Autodesk Inventor part; units mm, degrees
ref_plane "YZ Plane" through (0, 0, 0) normal (1, 0, 0) x (0, 1, 0)
ref_plane "XZ Plane" through (0, 0, 0) normal (0, 1, 0) x (-1, 0, 0)
ref_plane "XY Plane" through (0, 0, 0) normal (0, 0, 1) x (1, 0, 0)
sketch "Sketch1" plane through (0, 0, 0) normal (0, 0, 1) x (1, 0, 0)
  line L0 (-18.7833, 39.6114) -> (-18.7833, -39.6114)
  line L1 (-18.7833, -39.6114) -> (18.7833, -39.6114)
  line L2 (18.7833, -39.6114) -> (18.7833, 39.6114)
  line L3 (18.7833, 39.6114) -> (-18.7833, 39.6114)
  line L4 (-15.6083, 36.4364) -> (15.6083, 36.4364)
  line L5 (15.6083, 36.4364) -> (15.6083, -36.4364)
  line L6 (15.6083, -36.4364) -> (-15.6083, -36.4364)
  line L7 (-15.6083, -36.4364) -> (-15.6083, 36.4364)
  point P0 (0, 0)
extrude "Extrusion1" add sketch "Sketch1" along normal blind 3.175 contours L3 L2 L1 L0 | L4 L5 L6 L7
sketch "Sketch2" plane through (0, 0, 0) normal (0, 0, -1) x (-1, 0, 0)
  line L0 (-15.6083, -36.4364) -> (15.6083, -36.4364)
  line L1 (-15.6083, 36.4364) -> (-15.6083, -36.4364)
  line L2 (15.6083, 36.4364) -> (-15.6083, 36.4364)
  line L3 (15.6083, -36.4364) -> (15.6083, 36.4364)
  line L4 (-15.3543, 36.1824) -> (-15.3543, -36.1824)
  line L5 (-15.3543, -36.1824) -> (15.3543, -36.1824)
  line L6 (15.3543, -36.1824) -> (15.3543, 36.1824)
  line L7 (15.3543, 36.1824) -> (-15.3543, 36.1824)
  point P0 (0, 0)
  dimension "d2" = 0.254
extrude "Extrusion2" add sketch "Sketch2" along normal blind 1.5875 contours L7 L6 L5 L4
sketch "Sketch3" plane through (0, 0, -1.5875) normal (0, 0, -1) x (-1, 0, 0)
  line L0 (-15.3543, 36.1824) -> (-15.3543, -36.1824)
  line L1 (-15.3543, 36.1824) -> (-9.0043, 36.1824)
  line L2 (-9.0043, 36.1824) -> (-9.0043, 29.8324)
  line L3 (-9.0043, 29.8324) -> (-15.3543, 29.8324)
  line L4 (-15.3543, 29.8324) -> (-15.3543, 36.1824)
  line L5 (15.3543, 36.1824) -> (-15.3543, 36.1824)
  line L6 (15.3543, 36.1824) -> (9.0043, 36.1824)
  line L7 (9.0043, 36.1824) -> (9.0043, 29.8324)
  line L8 (9.0043, 29.8324) -> (15.3543, 29.8324)
  line L9 (15.3543, 29.8324) -> (15.3543, 36.1824)
  line L10 (-15.3543, -36.1824) -> (15.3543, -36.1824)
  line L11 (-15.3543, -36.1824) -> (-9.0043, -36.1824)
  line L12 (-9.0043, -36.1824) -> (-9.0043, -29.8324)
  line L13 (-9.0043, -29.8324) -> (-15.3543, -29.8324)
  line L14 (-15.3543, -29.8324) -> (-15.3543, -36.1824)
  line L15 (15.3543, 36.1824) -> (15.3543, -36.1824)
  line L16 (15.3543, -36.1824) -> (9.0043, -36.1824)
  line L17 (9.0043, -36.1824) -> (9.0043, -29.8324)
  line L18 (9.0043, -29.8324) -> (15.3543, -29.8324)
  line L19 (15.3543, -29.8324) -> (15.3543, -36.1824)
  point P0 (0, 0)
  dimension "d5" = 6.35
  dimension "d6" = 6.35
  dimension "d7" = 6.35
  dimension "d8" = 6.35
  dimension "d9" = 6.35
  dimension "d10" = 6.35
  dimension "d11" = 6.35
  dimension "d12" = 6.35
extrude "Extrusion3" add sketch "Sketch3" along normal blind 5.08 contours L1 L2 L3 L0 | L13 L12 L10 L0 | L5 L9 L8 L7 | L17 L18 L15 L10
sketch "Sketch4" plane through (15.3543, -36.1824, 0) normal (1, 0, 0) x (0, 0, -1)
  line L0 (6.6675, 66.0147) -> (6.6675, 72.3647)
  line L1 (0, 72.3647) -> (0, 0)
  line L2 (6.6675, 0) -> (6.6675, 6.35)
  line L3 (1.5875, 66.0147) -> (1.5875, 6.35)
  line L4 (0, 72.3647) -> (6.6675, 72.3647)
  line L5 (1.5875, 6.35) -> (6.6675, 6.35)
  line L6 (6.6675, 6.35) -> (6.6675, 0)
  line L7 (1.5875, 6.35) -> (6.6675, 0)
  line L8 (1.5875, 66.0147) -> (6.6675, 72.3647)
  point P0 (0, 36.1824)
  point P1 (4.1275, 3.175)
  point P2 (4.1275, 69.1897)
  point P3 (4.1275, 3.175)
  point P4 (4.1275, 69.1897)
sketch "Sketch5" plane through (-15.3543, -36.1824, 0) normal (-1, 0, 0) x (0, 0, 1)
  point P0 (0, 36.1824)
  point P1 (-4.1275, 69.1897)
  point P2 (-4.1275, 3.175)
hole "Hole1" at (15.3543, 33.0074, -4.1275) at (15.3543, -33.0074, -4.1275) direction (-1, 0, 0) diameter 3.556 depth 5.842 countersink diameter 3.81 countersink angle 82
hole "Hole2" at (-15.3543, 33.0074, -4.1275) at (-15.3543, -33.0074, -4.1275) direction (1, 0, 0) diameter 3.556 depth 5.842 countersink diameter 3.81 countersink angle 82
sketch "Sketch6" plane through (0, 0, 3.175) normal (0, 0, 1) x (1, 0, 0)
  line L0 (-8.6233, 0) -> (8.6233, 0) construction
  line L1 (-8.6233, 2.54) -> (8.6233, 2.54)
  line L2 (8.6233, -2.54) -> (-8.6233, -2.54)
  arc A0 (-8.6233, 2.54) -> (-8.6233, -2.54) centre (-8.6233, 0) ccw
  arc A1 (8.6233, -2.54) -> (8.6233, 2.54) centre (8.6233, 0) ccw
  line L3 (-18.7833, 39.6114) -> (-18.7833, -39.6114)
  line L4 (18.7833, -39.6114) -> (18.7833, 39.6114)
  line L5 (-18.7833, -39.6114) -> (18.7833, -39.6114)
  arc A2 (8.6233, 10.16) -> (8.6233, 15.24) centre (8.6233, 12.7) ccw
  line L6 (-8.6233, 15.24) -> (8.6233, 15.24)
  line L7 (8.6233, 10.16) -> (-8.6233, 10.16)
  arc A3 (-8.6233, 15.24) -> (-8.6233, 10.16) centre (-8.6233, 12.7) ccw
  arc A4 (8.6233, 22.86) -> (8.6233, 27.94) centre (8.6233, 25.4) ccw
  line L8 (-8.6233, 27.94) -> (8.6233, 27.94)
  line L9 (8.6233, 22.86) -> (-8.6233, 22.86)
  arc A5 (-8.6233, 27.94) -> (-8.6233, 22.86) centre (-8.6233, 25.4) ccw
  arc A6 (8.6233, -15.24) -> (8.6233, -10.16) centre (8.6233, -12.7) ccw
  line L10 (-8.6233, -10.16) -> (8.6233, -10.16)
  line L11 (8.6233, -15.24) -> (-8.6233, -15.24)
  arc A7 (-8.6233, -10.16) -> (-8.6233, -15.24) centre (-8.6233, -12.7) ccw
  arc A8 (8.6233, -2.54) -> (8.6233, 2.54) centre (8.6233, 0) ccw
  line L12 (-8.6233, 2.54) -> (8.6233, 2.54)
  line L13 (8.6233, -2.54) -> (-8.6233, -2.54)
  arc A9 (-8.6233, 2.54) -> (-8.6233, -2.54) centre (-8.6233, 0) ccw
  arc A10 (8.6233, 10.16) -> (8.6233, 15.24) centre (8.6233, 12.7) ccw
  line L14 (-8.6233, 15.24) -> (8.6233, 15.24)
  line L15 (8.6233, 10.16) -> (-8.6233, 10.16)
  arc A11 (-8.6233, 15.24) -> (-8.6233, 10.16) centre (-8.6233, 12.7) ccw
  arc A12 (8.6233, -27.94) -> (8.6233, -22.86) centre (8.6233, -25.4) ccw
  line L16 (-8.6233, -22.86) -> (8.6233, -22.86)
  line L17 (8.6233, -27.94) -> (-8.6233, -27.94)
  arc A13 (-8.6233, -22.86) -> (-8.6233, -27.94) centre (-8.6233, -25.4) ccw
  arc A14 (8.6233, -15.24) -> (8.6233, -10.16) centre (8.6233, -12.7) ccw
  line L18 (-8.6233, -10.16) -> (8.6233, -10.16)
  line L19 (8.6233, -15.24) -> (-8.6233, -15.24)
  arc A15 (-8.6233, -10.16) -> (-8.6233, -15.24) centre (-8.6233, -12.7) ccw
  arc A16 (8.6233, -2.54) -> (8.6233, 2.54) centre (8.6233, 0) ccw
  line L20 (-8.6233, 2.54) -> (8.6233, 2.54)
  line L21 (8.6233, -2.54) -> (-8.6233, -2.54)
  arc A17 (-8.6233, 2.54) -> (-8.6233, -2.54) centre (-8.6233, 0) ccw
  circle A18 centre (0, 12.7) radius 2.54
  circle A19 centre (0, 0) radius 2.54
  point P0 (0, 0)
  point P1 (0, 10.16)
  point P2 (0, 15.24)
  point P3 (0, 2.54)
  point P4 (0, -2.54)
  dimension "d29" = 10.16
  dimension "d30" = 10.16
  dimension "d31" = 2.54
  dimension "d35" = 12.7
  dimension "d38" = 12.7
extrude "Extrusion4" cut sketch "Sketch6" against normal up to surface (4.7625 mm away) contours L1 A1 L2 A19 | A19 | L7 A18 L6 A2 | A18 | L9 A5 L8 A4 | L11 A7 L10 A6 | L17 A13 L16 A12
sketch "Sketch7" plane through (0, 0, 3.175) normal (0, 0, 1) x (1, 0, 0)
  circle A0 centre (-7.3787, 6.5914) radius 5.715
  line L0 (18.7833, 39.6114) -> (-18.7833, 39.6114)
  line L1 (-18.7833, 39.6114) -> (-18.7833, -39.6114)
  line L2 (18.7833, -39.6114) -> (18.7833, 39.6114)
  point P0 (0, 0)
  dimension "d43" = 11.43
  dimension "d44" = 33.02
  dimension "d46" = 26.162
extrude "Extrusion5" cut sketch "Sketch7" against normal up to surface (4.7625 mm away)
properties part number "SENSOR_TOP" material "PC/ABS Plastic"
Here's how the part is built. I have some questions about the finished solid (model axes, mm). A direction names the side the tool comes from. Coordinates: 2 decimals unless noted, no trailing zeros. Write each loop counter-clockwise with the first axis right and the second up, starting at its lowest first coordinate (ties: lowest second). Pieces come first, ordered by that corner, then holes. Notation, with made-up numbers: (6, 14) - (31, 14) arc R15 ccw to (31, 20) - close; hole circle Ø2 at (5.5, 50.5). An arc over 180 degrees is marked (long way). One line per item, written item: value.
1) We'd pull the mould along X, two halves only. Please class faces 5 (the flat face through (4, 10.16, 1)), 6 (the flat face through (-12, -33, -6.668)), 7 (the flat face through (-9.004, 33, -4)): pulls with the +X half, pulls with the -X half, needs draft (parallel to the pull), parting line crosses it, or undercut.
Model answer:
face 5: undercut
face 6: needs draft
face 7: undercut
2) Suppose I cut it at D-D on y = 25.4. Write out the boundary of the cut face in (x, z) (1 decimal).
Model answer:
outline: (-18.8, 0) - (-15.4, 0) - (-15.4, -1.6) - (-11.2, -1.6) - (-11.2, 3.2) - (-18.8, 3.2) - close; (11.2, -1.6) - (15.4, -1.6) - (15.4, 0) - (18.8, 0) - (18.8, 3.2) - (11.2, 3.2) - close
3) I need wall thicknesses on line 1 along Y through (x, z) = (-14, -4); line 2 along Y through (x, z) = (6, 0.5); line 3 along Y through (x, z) = (15, -3). Which ranges of each line are inside material? Lowest first, please.
Model answer:
line 1: y = -36.18 to -34.78, -31.23 to -29.83, 29.83 to 31.23, 34.78 to 36.18
line 2: y = -39.61 to -27.94, -22.86 to -15.24, -10.16 to -2.54, 2.54 to 10.16, 15.24 to 22.86, 27.94 to 39.61
line 3: y = -36.18 to -34.38, -31.63 to -29.83, 29.83 to 31.63, 34.38 to 36.18
4) Suppose I cut it at C-C on z = 1.5. Write out the boundary of the cut face in (x, y) (3 decimals), and give its area (3 significant figures).
Model answer:
outline: (-18.783, -39.611) - (18.783, -39.611) - (18.783, 39.611) - (-18.783, 39.611) - close; hole circle Ø11.43 at (-7.379, 6.591); hole (-8.623, -27.94) - (8.623, -27.94) arc R2.54 ccw to (8.623, -22.86) - (-8.623, -22.86) arc R2.54 ccw to start; hole (-8.623, -15.24) - (8.623, -15.24) arc R2.54 ccw to (8.623, -10.16) - (-8.623, -10.16) arc R2.54 ccw to start; hole (-8.623, 22.86) - (8.623, 22.86) arc R2.54 ccw to (8.623, 27.94) - (-8.623, 27.94) arc R2.54 ccw to start; hole (0, -2.54) - (8.623, -2.54) arc R2.54 ccw to (8.623, 2.54) - (0, 2.54) arc R2.54 ccw to start; hole (0, 10.16) - (8.623, 10.16) arc R2.54 ccw to (8.623, 15.24) - (0, 15.24) arc R2.54 ccw to start
area: 2,420 mm²
5) I'm going to push flat-ended pins straight in: P1, Ø4, axis at y = -8, z = -4, coming from the +X side; P2, Ø5.5, axis at y = -33.01, z = -4.13, coming from the -X side; P3, Ø2.5, axis at x = -12, z = -3.5, coming from the -Y side; P4, Ø4, axis at y = 33.5, z = -3.5, coming from the +X side. Where does each tip first touch, or does it pass through?
Model answer:
P1: passes through
P2: stops at x = -15.35
P3: stops at y = -36.18
P4: stops at x = 15.35
6) Suppose I cut it at A-A on y = 0. Write out the boundary of the cut face in (x, z) (1 decimal).
Model answer:
outline: (-18.8, 0) - (-15.4, 0) - (-15.4, -1.6) - (-2.5, -1.6) - (-2.5, 3.2) - (-18.8, 3.2) - close; (11.2, -1.6) - (15.4, -1.6) - (15.4, 0) - (18.8, 0) - (18.8, 3.2) - (11.2, 3.2) - close
7) On a 3-axis mill with a long thin cutter (end or side, diameter ignored), from which of +Z, -Z, +X, -X, +Y, -Y can I reach the whole of each face in a straight line? I mean faces 1 (the cylindrical face through (-12.32, 31.245, -4.359)), 2 (the flat face through (-12, 29.832, -4)), 3 (the flat face through (0, 36.182, -1)), 4 (the cylindrical face through (11.163, -0.056, 0.827)). Say none if no direction works.
Model answer:
face 1: -X
face 2: -Z, +X, -X
face 3: -Z, +X, -X, +Y
face 4: +Z, -Z
8) Suppose I cut it at B-B on x = 13. Write out the boundary of the cut face in (y, z) (1 decimal), and give its area (3 significant figures).
Model answer:
outline: (-39.6, 0) - (-36.2, 0) - (-36.2, -6.7) - (-29.8, -6.7) - (-29.8, -1.6) - (29.8, -1.6) - (29.8, -6.7) - (36.2, -6.7) - (36.2, 0) - (39.6, 0) - (39.6, 3.2) - (-39.6, 3.2) - close; hole circle Ø3.6 at (-33, -4.1); hole circle Ø3.6 at (33, -4.1)
area: 411 mm²
